Work out the finished part from the listing and answer in its coordinate system (mm). Face numbers are marked on the shaded views. A direction names the side the tool comes from. Round coordinates to 2 decimals unless told otherwise and drop trailing zeros. Order: outer loops, then holes, each group sorted by start corner. A loop starts at its lowest first (then second) coordinate and runs counter-clockwise, first axis right, second up. Notation, with made-up numbers: (63, 40.25) -> (68, 40.25) arc R37 cw to (68, 76.25) -> close; hole circle Ø2 at (68, -1). An arc over 180 degrees is marked (long way). Use one line per item in the form item = value.
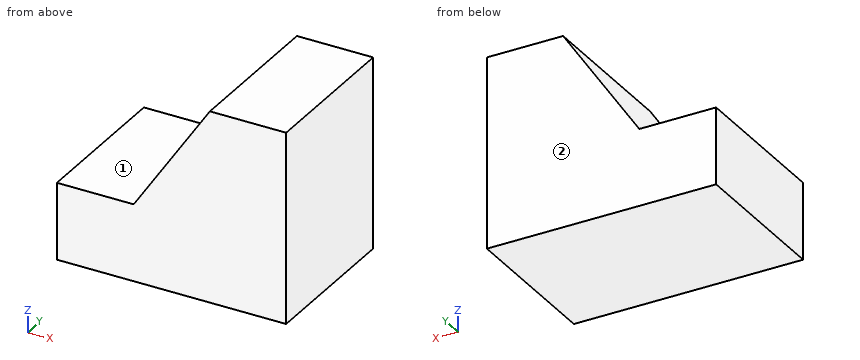
```python
from build123d import *

# Parameters (mm, degrees)
F0_W     = 38.1
F0_H     = 31.75
F1_DEPTH = 25.4
F3_DEPTH = 25.4
F5_DEPTH = 25.401


with BuildPart() as f1:
    # F0 (on Front) → F1 (new body)
    with BuildSketch(Plane.XZ):
        with Locations((19.05, 15.875)):
            Rectangle(F0_W, F0_H)
    extrude(amount=F1_DEPTH)

    # F2 (on Front) → F3 (cut)
    with BuildSketch(Plane.XZ):
        Polygon((23.017952, 8.342751), (23.017952, 31.260189), (0, 12.564384), (0, 8.342751), align=None)
    extrude(amount=-F3_DEPTH, mode=Mode.SUBTRACT)

    # F4 (on face) → F5 (cut, through all)
    with BuildSketch(Plane.XZ.offset(25.4)):
        Polygon((0, 31.75), (0, 12.765414), (12.765414, 12.765414), (25.430316, 31.75), align=None)
    extrude(amount=-F5_DEPTH, mode=Mode.SUBTRACT)


solid = f1.part
```
Item 1: For the marked faces 1 and 2, determine the directions among +Z, -Z, +X, -X, +Y, -Y from which every point of the face is accessible in a straight line to the end or side of a thin tool.
Findings:
face_1 = +Z, -X, +Y, -Y
face_2 = +Z, -Z, +X, -X, +Y
Item 2: The part is cut by section A-A, the plane y = -13.25. Give the vertices of the cut face in (x, z).
Findings:
outline = (0, 0) -> (38.1, 0) -> (38.1, 31.75) -> (25.43, 31.75) -> (12.77, 12.77) -> (0, 12.77) -> close
Item 3: Consider line 1 along Z through (x, y) = (11, -3.75); line 2 along X through (y, z) = (-16, 13); line 3 along X through (y, z) = (-21, 14). Determine where each line is inside the solid, lowest interval first.
Findings:
line_1 = 0 to 12.77
line_2 = 12.92 to 38.1
line_3 = 13.59 to 38.1
Item 4: The part is cut by section B-B, the plane x = 20. Give the vertices of the cut face in (y, z).
Findings:
outline = (-25.4, 0) -> (0, 0) -> (0, 23.61) -> (-25.4, 23.61) -> close
Item 5: Flat-ended cylindrical pins translate along their axes: P1, Ø1, axis at x = 4.5, y = -19, coming from the +Z side; P2, Ø6, axis at y = -20, z = 26.5, coming from the -X side; P3, Ø2, axis at y = -8.5, z = 19, coming from the -X side. Find the tip coordinate at first contact, or state that the pin passes through.
Findings:
P1 = 12.77
P2 = 19.93
P3 = 16.26
Item 6: The part is cut by section C-C, the plane z = 15.5. Give the vertices of the cut face in (x, y).
Findings:
outline = (14.59, -25.4) -> (38.1, -25.4) -> (38.1, 0) -> (14.59, 0) -> close
